```python
from build123d import *

# Parameters (mm, degrees)
SKETCH1_W               = 254
SKETCH1_H               = 254
PLATFORM_BASE_DEPTH     = 7.62
SKETCH7_W               = 76.2
SKETCH7_H               = 101.6
CUT_EXTRUDE4_DEPTH      = 180.766694357
CORNER_ROUNDING_R       = 25.4
SKETCH6_W               = 12.7
SKETCH6_H               = 7.62
CUT_EXTRUDE3_DEPTH      = 180.766694357
MIRROR6_COPY_1_SKETCH_W = 12.7
MIRROR6_COPY_1_SKETCH_H = 7.62
MIRROR6_COPY_1_DEPTH    = 180.766694357


with BuildPart() as part:
    # Sketch1 → Platform-Base (new body)
    with BuildSketch(Plane(origin=(0, 0, 0), x_dir=(1, 0, 0), z_dir=(0, 1, 0))):
        Rectangle(SKETCH1_W, SKETCH1_H)
    extrude(amount=PLATFORM_BASE_DEPTH)

    # Sketch7 → Cut-Extrude4 (cut, through all)
    with BuildSketch(Plane(origin=(0, 7.62, 0), x_dir=(1, 0, 0), z_dir=(0, 1, 0))):
        with Locations((0, -55.88)):
            Rectangle(SKETCH7_W, SKETCH7_H)
    cut_extrude4 = extrude(amount=-CUT_EXTRUDE4_DEPTH, mode=Mode.SUBTRACT)

    # Corner-Rounding
    corner_rounding_edges = [part.edges().sort_by_distance(p)[0] for p in [
        (127, 3.81, 127),
        (-127, 3.81, 127),
        (-127, 3.81, -127),
        (127, 3.81, -127),
    ]]
    fillet(corner_rounding_edges, radius=CORNER_ROUNDING_R)

    # Sketch6 → Cut-Extrude3 (cut, through all)
    with BuildSketch(Plane(origin=(0, 7.62, 0), x_dir=(1, 0, 0), z_dir=(0, 1, 0))):
        with Locations((-76.2, -123.19)):
            Rectangle(SKETCH6_W, SKETCH6_H)
    cut_extrude3 = extrude(amount=-CUT_EXTRUDE3_DEPTH, mode=Mode.SUBTRACT)

    # Mirror4: Cut-Extrude3 across plane
    add(cut_extrude3.mirror(Plane.XY), mode=Mode.SUBTRACT)

    # Mirror5: Cut-Extrude4 across plane
    add(cut_extrude4.mirror(Plane.XY), mode=Mode.SUBTRACT)

    # Mirror6: Cut-Extrude3 across plane
    add(cut_extrude3.mirror(Plane.ZY), mode=Mode.SUBTRACT)

    # Mirror6 copy 1 sketch → Mirror6 copy 1 (cut, through all)
    with BuildSketch(Plane(origin=(0, 7.62, 0), x_dir=(-1, 0, 0), z_dir=(0, 1, 0))):
        with Locations((-76.2, -123.19)):
            Rectangle(MIRROR6_COPY_1_SKETCH_W, MIRROR6_COPY_1_SKETCH_H)
    extrude(amount=-MIRROR6_COPY_1_DEPTH, mode=Mode.SUBTRACT)


solid = part.part
```
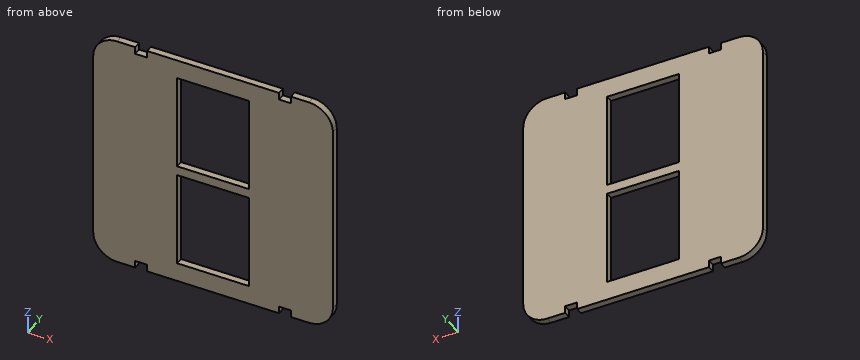
Geometry check sheet. Reference: the model listing, model coordinates, mm. Give positions to 0.01 mm unless a question says otherwise; leave off trailing zeros. Loops run counter-clockwise (first coordinate to the right, second up) from the corner with the lowest first, then second, coordinate; pieces in that order, holes last. Notation, with made-up numbers: M -27,75.5 L 15,75.5 A5 ccw 15,82.5 Z; hole C -21.5,-36 d8. An arc over 180 degrees is marked long. Write item = value, one per line.
(1) Material ranges on line 1 (Z direction, x = -22.5, y = 3.75); line 2 (X direction, y = 4.75, z = -13); line 3 (Z direction, x = 77.5, y = 2.5), recorded low to high. Write a range as [from, to].
Answer below:
line_1 = [-127, -106.68], [-5.08, 5.08], [106.68, 127]
line_2 = [-127, -38.1], [38.1, 127]
line_3 = [-119.38, 119.38]
(2) Sectioned sample at A-A, the plane z = 33. Record the cut outline in (x, y), plus the area to 3 significant figures.
Answer below:
outline = M -127,0 L -38.1,0 L -38.1,7.62 L -127,7.62 Z; M 38.1,0 L 127,0 L 127,7.62 L 38.1,7.62 Z
area = 1,350 mm2
(3) Sectioned sample at B-B, the plane x = -17. Record the cut outline in (y, z).
Answer below:
outline = M 0,-127 L 7.62,-127 L 7.62,-106.68 L 0,-106.68 Z; M 0,-5.08 L 7.62,-5.08 L 7.62,5.08 L 0,5.08 Z; M 0,106.68 L 7.62,106.68 L 7.62,127 L 0,127 Z
(4) Sectioned sample at C-C, the plane y = 5.25. State how many separate pieces and enclosed holes the cut face has, plus the area to 3 significant figures.
Answer below:
separate_pieces = 1
enclosed_holes = 2
area = 48,100 mm2
(5) Gauge pin test, flat ends, axial feed: pin 1 Ø4 at (y, z) = (2, -123.5) entering from +X; pin 2 Ø4 at (y, z) = (3.5, 122.5) entering from -X; pin 3 Ø4 at (y, z) = (5, 122) entering from +X. Record the tip position at first contact, or that the pin passes through.
Answer below:
pin_1 = 117.38
pin_2 = -118.57
pin_3 = 119.11
